Source: CAD feature listing. Evaluate the final solid. Frame: model axes, mm. A direction names the side the tool comes from. Coordinates: 2 decimals unless noted, no trailing zeros. Order: outer loops, then holes, each group sorted by start corner. A loop starts at its lowest first (then second) coordinate and runs counter-clockwise, first axis right, second up.
Autodesk Fusion 360 part; units mm, degrees
sketch "Sketch1" plane through (0, 0, 0) normal (0, 0, 1) x (1, 0, 0)
sketch "Sketch2" plane through (0, 0, 0) normal (0, 0, 1) x (1, 0, 0)
  line L0 (0, 0) -> (33, 0)
  line L1 (33, 0) -> (33, 33)
  line L2 (33, 33) -> (0, 33)
  line L3 (0, 33) -> (0, 0)
  arc A0 (33, 0) -> (0, 33) centre (-20.6429, -20.6429) ccw
  dimension "d1" = 33
  dimension "d2" = 33
extrude "Extrude1" add sketch "Sketch2" along normal blind 4.5 contours L0 L3 A0
move_face "OffsetFaces1" offset 1 3 faces at (11, 0, 1.5) (0, 22, 1.5) (21.8433, 18.069, 3)
extrude "Extrude2" cut sketch "Sketch2" along normal blind 3 from surface at 1.5 contours L0 L3 A0
fillet "Fillet1" radius 1 3 edges at (-1, -1, 2.25) (34.4371, -1, 2.25) (-1, 34.4371, 2.25)
chamfer "Chamfer1" distance 0.45 angle 45 3 edges at (0, 16.5, 4.5) (20, 20, 4.5) (16.5, 0, 4.5)
1. Access query for faces 4 (the face through (13, 13, 1.5)), 5 (the face through (33.8, -0.6, 2.2)). Directions: +Z, -Z, +X, -X, +Y, -Y. A direction counts if a zero-diameter tool reaches every point of the face in a straight line with its end or side. Return the directions, or none.
Findings:
face 4: +Z
face 5: +Z, -Z, +X
2. Pin query (flat end, axial travel): P1, Ø2, axis at x = 3.5, y = 17.5, coming from the +Z side; P2, Ø1.3, axis at y = 16.5, z = 2.5, coming from the +X side; P3, Ø2, axis at x = 27.5, z = 2, coming from the +Y side. Return the tip coordinate at first contact, or that it passes through.
Findings:
P1: stops at z = 1.5
P2: stops at x = 25.05
P3: stops at y = 13.96
3. Draft query along X for faces 1 (the face through (20, 20, 3)), 2 (the face through (19, 22, 4.5)), 3 (the face through (20.46, 20.95, 2.22)). Return one class per face: released by +X, released by -X, zero draft, split by the parting line, or undercut.
Findings:
face 1: undercut
face 2: zero draft
face 3: released by +X
4. Ray query, line 1 (Y direction, x = 16, z = 3.35); line 2 (Z direction, x = 9.5, y = 27.5); line 3 (Y direction, x = 11, z = 2.9). Return the intervals inside material, ascending.
Findings:
line 1: y = -1 to 0, 23.64 to 24.93
line 2: z = 0 to 1.5
line 3: y = -1 to 0, 27.34 to 28.53
5. Section query A-A on z = 2.45. Return loops of the section in (x, y).
Findings:
outline: (-1, 0) arc R1 ccw to (0, -1) - (33, -1) arc R1 ccw to (33.93, 0.36) arc R58.48 ccw to (0.36, 33.93) arc R1 ccw to (-1, 33) - close; hole (0, 0) - (33, 0) arc R57.48 ccw to (0, 33) - close
